Here's how the part is built. I have some questions about the finished solid (model axes, mm). A direction names the side the tool comes from. Coordinates: 2 decimals unless noted, no trailing zeros. Write each loop counter-clockwise with the first axis right and the second up, starting at its lowest first coordinate (ties: lowest second). Pieces come first, ordered by that corner, then holes.
Autodesk Inventor part; units mm, degrees
ref_plane "YZ Plane" through (0, 0, 0) normal (1, 0, 0) x (0, 1, 0)
ref_plane "XZ Plane" through (0, 0, 0) normal (0, 1, 0) x (-1, 0, 0)
ref_plane "XY Plane" through (0, 0, 0) normal (0, 0, 1) x (1, 0, 0)
sketch "Sketch1" plane through (0, 0, 0) normal (0, 0, 1) x (1, 0, 0)
  circle A0 centre (0, 0) radius 50
  line L0 (0, 0) -> (0, 20) construction
  line L1 (2.5, 15) -> (97.5, 15)
  line L2 (97.5, 15) -> (97.5, -15)
  line L3 (97.5, -15) -> (2.5, -15)
  line L4 (2.5, -15) -> (2.5, 15)
  line L5 (2.5, 15) -> (97.5, -15) construction
  line L6 (97.5, 15) -> (2.5, -15) construction
  line L7 (40, 5) -> (60, 5)
  line L8 (60, 5) -> (60, -5)
  line L9 (60, -5) -> (40, -5)
  line L10 (40, -5) -> (40, 5)
  line L11 (40, 5) -> (60, -5) construction
  line L12 (60, 5) -> (40, -5) construction
  line L13 (60, 5) -> (60, 15)
  line L14 (60, -5) -> (60, -15)
  line L15 (-2.5, 15) -> (-97.5, 15)
  line L16 (-97.5, 15) -> (-97.5, -15)
  line L17 (-97.5, -15) -> (-2.5, -15)
  line L18 (-2.5, -15) -> (-2.5, 15)
  line L19 (-2.5, 15) -> (-97.5, -15) construction
  line L20 (-97.5, 15) -> (-2.5, -15) construction
  line L21 (-40, 5) -> (-60, 5)
  line L22 (-60, 5) -> (-60, -5)
  line L23 (-60, -5) -> (-40, -5)
  line L24 (-40, -5) -> (-40, 5)
  line L25 (-40, 5) -> (-60, -5) construction
  line L26 (-60, 5) -> (-40, -5) construction
  line L27 (-60, 5) -> (-60, 15)
  line L28 (-60, -5) -> (-60, -15)
  point P0 (50, 0)
  point P1 (50, 0)
  point P2 (-50, 0)
  point P3 (-50, 0)
  point P4 (49.7494, 5)
  point P5 (49.7494, -5)
  point P6 (-49.7494, -5)
  point P7 (-49.7494, 5)
  dimension "d0" = 100
  dimension "d3" = 20
  dimension "d17" = 95
  dimension "d18" = 30
  dimension "d19" = 20
  dimension "d20" = 10
extrude "Extrusion1" add sketch "Sketch1" along normal blind 5 contours A0 L9 L10 L7 | A0 L7 L8 L9 | L7 L10 L9 A0 L3 L4 L1 | L1 L4 L3 A0 L17 L18 L15 | L13 L1 L2 L3 L14 L8 | L15 L18 L17 A0 L23 L24 L21 | L21 L24 L23 A0 | A0 L23 L22 L21 | L27 L22 L28 L17 L16 L15
sketch "Sketch2" plane through (0, 0, 5) normal (0, 0, 1) x (1, 0, 0)
  line L0 (0, 0) -> (-77.5, 0) construction
  circle A0 centre (-77.5, 0) radius 5.25
  line L1 (0, 0) -> (0, 20) construction
  circle A1 centre (-77.5, 0) radius 8
  circle A2 centre (-69.5, 0) radius 1.75
  circle A3 centre (-77.5, 8) radius 1.75
  circle A4 centre (-85.5, 0) radius 1.75
  circle A5 centre (-77.5, -8) radius 1.75
  circle A6 centre (77.5, 0) radius 12
  line L2 (65, 12.5) -> (90, 12.5)
  line L3 (90, 12.5) -> (90, -12.5)
  line L4 (90, -12.5) -> (65, -12.5)
  line L5 (65, -12.5) -> (65, 12.5)
  line L6 (65, 12.5) -> (90, -12.5) construction
  line L7 (90, 12.5) -> (65, -12.5) construction
  line L8 (90, 12.5) -> (65, -12.5)
  circle A7 centre (85.9853, 8.4853) radius 1.75
  circle A8 centre (69.0147, 8.4853) radius 1.75
  circle A9 centre (69.0147, -8.4853) radius 1.75
  circle A10 centre (85.9853, -8.4853) radius 1.75
  circle A11 centre (77.5, 0) radius 7.6
  dimension "d26" = 16
  dimension "d70" = 24
  dimension "d6" = 77.5
  dimension "d7" = 10.5
  dimension "d8" = 20
  dimension "d27" = 3.5
  dimension "d30" = 360
  dimension "d71" = 25
  dimension "d72" = 25
  dimension "d73" = 3.5
  dimension "d76" = 360
  dimension "d78" = 15.2
extrude "Extrusion2" cut sketch "Sketch2" against normal blind 7 contours A0 | A1 A2 | A1 A2 | A3 A1 | A1 A3 | A5 A1 | A1 A5 | A4 A1 | A1 A4 | A7 L8 A6 | A6 L8 A7 | A10 A6 | A6 A10 | L8 A7 A6 | A6 A7 L8 | A11 L8 | L8 A11 | A9 L8 A6 | A6 L8 A9 | A8 A6 | A6 A8 | L8 A9 A6 | A6 A9 L8
fillet "Fillet1" radius 3 16 edges at (-60, 5, 2.5) (-60, 15, 2.5) (-49.7494, 5, 2.5) (-60, -5, 2.5) (-60, -15, 2.5) (-49.7494, -5, 2.5) (-97.5, -15, 2.5) (-97.5, 15, 2.5) (97.5, 15, 2.5) (97.5, -15, 2.5) (60, -15, 2.5) (60, 15, 2.5) (60, -5, 2.5) (60, 5, 2.5) (49.7494, 5, 2.5) (49.7494, -5, 2.5)
sketch "Sketch4" plane through (0, 0, 5) normal (0, 0, 1) x (1, 0, 0)
  line L0 (-7.5, 22.5) -> (7.5, 22.5)
  line L1 (7.5, 22.5) -> (7.5, -22.5)
  line L2 (7.5, -22.5) -> (-7.5, -22.5)
  line L3 (-7.5, -22.5) -> (-7.5, 22.5)
  line L4 (-7.5, 22.5) -> (7.5, -22.5) construction
  line L5 (7.5, 22.5) -> (-7.5, -22.5) construction
  circle A0 centre (0, -22.5) radius 7.5
  circle A1 centre (0, 22.5) radius 7.5
  point P0 (0, 0)
  point P1 (7.5, 22.5)
  dimension "d79" = 15
  dimension "d80" = 45
  dimension "d81" = 15
  dimension "d82" = 15
extrude "Extrusion3" cut sketch "Sketch4" against normal blind 10
properties part number "TAPA OPCION 3"
1. Thinking about a two-plate mould opening in X: for faces 1 (the face through (20, 1, 5)), 2 (the face through (55, -5, 2)), 3 (the face through (-97.5, 0, 2)), which applies, pulls with the +X half, pulls with the -X half, needs draft (parallel to the pull), parting line crosses it, or undercut?
2. On a 3-axis mill with a long thin cutter (end or side, diameter ignored), from which of +Z, -Z, +X, -X, +Y, -Y can I reach the whole of each face in a straight line? I mean faces 4 (the face through (79, 15, 2)), 5 (the face through (0, 30, 3)), 6 (the face through (60, 10, 2)), 7 (the face through (-79, -15, 2)). Say none if no direction works.
3. For pin 1 Ø2.5 at (x, z) = (-86, 3.5) entering from +Y; pin 2 Ø2.5 at (x, z) = (53.5, 1.5) entering from +Y, each with a flat end and sliding along its axis, tell me the tip position at first contact or that it passes through.
4. I want a section at D-D (x = -39.5). List the corners of the cut face in (y, z) for me, then the cut area to 3 significant figures.
5. If I drill on line 1 (Y direction, x = -77.5, z = 1.7); line 2 (X direction, y = -11.5, z = 3.15); line 3 (X direction, y = 2, z = 0.85), over which ranges is the centre line in solid material (lowest first)?
6. I want a section at C-C (z = 4.1). State how many separate pieces and enclosed holes the cut face has, then the cut area to 3 significant figures.
7. I want a section at B-B (x = 77.5). List the corners of the cut face in (y, z) for me, then the cut area to 3 significant figures.
8. I want a section at A-A (x = 0). List the corners of the cut face in (y, z) for me.
Response values:
1. face 1: needs draft
1. face 2: undercut
1. face 3: pulls with the -X half
2. face 4: +Z, -Z, +X, +Y
2. face 5: +Z, -Z
2. face 6: +Z, -Z, +Y
2. face 7: +Z, -Z, -X, -Y
3. pin 1: stops at y = 15
3. pin 2: stops at y = 5
4. outline: (-30.66, 0) - (30.66, 0) - (30.66, 5) - (-30.66, 5) - close
4. area: 307 mm2
5. line 1: y = -15 to -9.75, -6.25 to -5.25, 5.25 to 6.25, 9.75 to 15
5. line 2: x = -97.5 to -60, -48.66 to -7.5, 7.5 to 48.66, 60 to 97.5
5. line 3: x = -97.5 to -82.35, -72.65 to -7.5, 7.5 to 70.17, 84.83 to 97.5
6. separate pieces: 1
6. enclosed holes: 11
6. area: 9,110 mm2
7. outline: (-15, 0) - (-7.6, 0) - (-7.6, 5) - (-15, 5) - close; (7.6, 0) - (15, 0) - (15, 5) - (7.6, 5) - close
7. area: 74.0 mm2
8. outline: (-50, 0) - (-30, 0) - (-30, 5) - (-50, 5) - close; (30, 0) - (50, 0) - (50, 5) - (30, 5) - close
